Geometry check sheet. Reference: the model listing, model coordinates, mm. A direction names the side the tool comes from. Round coordinates to 2 decimals unless told otherwise and drop trailing zeros. Write each loop counter-clockwise with the first axis right and the second up, starting at its lowest first coordinate (ties: lowest second). Pieces come first, ordered by that corner, then holes. Notation, with made-up numbers: M 47,31.25 L 85,31.25 A21 cw 85,43.25 Z; hole C 71,-10 d10. An arc over 180 degrees is marked long. Answer in a Markdown table with one row per item. Add a question column.
from build123d import *

# Parameters (mm, degrees)
ESQUISSE1_R    = 6
CORP_DEPTH     = 8.2
ESQUISSE2_R    = 1.25
TROU_SON_DEPTH = 1
ESQUISSE3_R    = 0.4
PINS_DEPTH     = 3
CONG_1_R       = 0.6
ESQUISSE4_R    = 1.25
PLUS_DEPTH     = 0.1


with BuildPart() as part:
    # Esquisse1 → corp (new body)
    with BuildSketch(Plane.XY):
        Circle(ESQUISSE1_R)
    extrude(amount=CORP_DEPTH)

    # Esquisse2 → trou son (cut)
    with BuildSketch(Plane.XY.offset(8.2)):
        Circle(ESQUISSE2_R)
    extrude(amount=-TROU_SON_DEPTH, mode=Mode.SUBTRACT)

    # Esquisse3 → pins (add)
    with BuildSketch(Plane.XY):
        with Locations((3.3, 0)):
            Circle(ESQUISSE3_R)
        with Locations(Location((-3.3, 0, 0), (0, 0, 180))):
            Circle(ESQUISSE3_R)
    extrude(amount=-PINS_DEPTH)

    # Congé1
    cong_1_edges = [part.edges().sort_by_distance(p)[0] for p in [
        (-6, 0, 8.2),
    ]]
    fillet(cong_1_edges, radius=CONG_1_R)

    # Esquisse4 → plus (cut)
    with BuildSketch(Plane.XY.offset(8.2)):
        with Locations((-3.625, 0)):
            Circle(ESQUISSE4_R)
        Polygon((-2.625, -0.125), (-2.625, 0.125), (-3.5, 0.125), (-3.5, 1), (-3.75, 1), (-3.75, 0.125), (-4.625, 0.125), (-4.625, -0.125), (-3.75, -0.125), (-3.75, -1), (-3.5, -1), (-3.5, -0.125), align=None, mode=Mode.SUBTRACT)
    extrude(amount=-PLUS_DEPTH, mode=Mode.SUBTRACT)


solid = part.part
Item 1: Section check A-A, the plane z = -2.25. Record the boundary of the cut face in (x, y), and give its area (3 significant figures).
Item 2: Section check C-C, the plane z = 3.5. Record the boundary of the cut face in (x, y).
Item 3: Mould release check, pull along Y, two halves, no side actions. Record for faces 1 (the flat face through (-3.92, 0.3, 8.1)), 2 (the flat face through (1, -1, 8.2)), 3 (the cylindrical face through (-6, 0, 4)): +Y half, -Y half, draft (parallel to the pull), parting line (faces both ways), or undercut.
Item 4: Gauge pin test, flat ends, axial feed: pin 1 Ø5 at (x, z) = (3, -0.5) entering from -Y; pin 2 Ø2 at (x, z) = (3, 4) entering from +Y; pin 3 Ø0.8 at (x, y) = (0, 0.5) entering from +Z. Record the tip position at first contact, or that the pin passes through.
Item 5: Scan lines: probe 1 along Z at (x, y) = (1.75, -3.75); probe 2 along Y at (x, z) = (0, 7.7); probe 3 along Y at (x, z) = (-4, 0.5). Record each from-to range of solid material in increasing order. Write a range as from..to.
Item 6: Access from +Z, -Z, +X, -X, +Y, -Y to the whole of each face (thin tool, end or side, straight path). Record for faces 4 (the flat face through (-3.6, 0, 8.2)), 5 (the cylindrical face through (-0.27, -1.22, 7.71)).
Item 7: Section check B-B, the plane x = 0. Record the boundary of the cut face in (y, z), and give its area (3 significant figures).
Result sheet:
| question | item | result |
|---|---|---|
| 1 | outline | C -3.3,0 d0.8; C 3.3,0 d0.8 |
| 1 | area | 1.01 mm^2 |
| 2 | outline | C 0,0 d12 |
| 3 | face 1 | undercut |
| 3 | face 2 | draft |
| 3 | face 3 | parting line |
| 4 | pin 1 | stops at y = -5.97 |
| 4 | pin 2 | stops at y = 5.66 |
| 4 | pin 3 | stops at z = 7.2 |
| 5 | probe 1 | z = 0..8.2 |
| 5 | probe 2 | y = -5.99..-1.25, 1.25..5.99 |
| 5 | probe 3 | y = -4.47..4.47 |
| 6 | face 4 | +Z, +X, -X, +Y, -Y |
| 6 | face 5 | +Z |
| 7 | outline | M -6,0 L 6,0 L 6,7.6 A0.6 ccw 5.4,8.2 L 1.25,8.2 L 1.25,7.2 L -1.25,7.2 L -1.25,8.2 L -5.4,8.2 A0.6 ccw -6,7.6 Z |
| 7 | area | 95.7 mm^2 |
